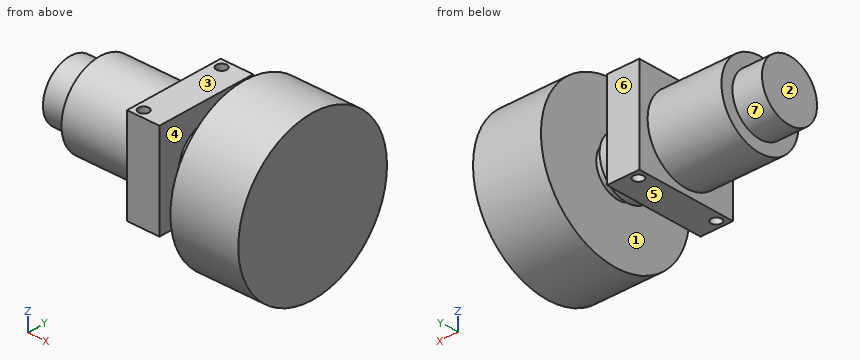
from build123d import *

# Parameters (mm, degrees)
SKETCH_R          = 14
PAD_DEPTH         = 25
SKETCH001_W       = 34
SKETCH001_H       = 32
PAD001_DEPTH      = 11
SKETCH002_R       = 10
PAD002_DEPTH      = 9
SKETCH003_R       = 8
PAD003_DEPTH      = 3
PAD004_DEPTH      = 12
SKETCH005_R       = 1.75
POCKET_DEPTH      = 100
SKETCH006_R       = 27
PAD005_DEPTH      = 12
PAD005_DEPTH_BACK = 11
SKETCH007_R       = 10
PAD006_DEPTH      = 10


with BuildPart() as part:
    # Sketch → Pad (new body)
    with BuildSketch(Plane.YZ):
        Circle(SKETCH_R)
    extrude(amount=-PAD_DEPTH)

    # Sketch001 (on Face2 of Pad) → Pad001 (join)
    with BuildSketch(Plane.YZ):
        Rectangle(SKETCH001_W, SKETCH001_H)
    extrude(amount=PAD001_DEPTH)

    # Sketch002 (on Face5 of Pad001) → Pad002 (join)
    with BuildSketch(Plane.YZ.offset(11)):
        Circle(SKETCH002_R)
    extrude(amount=PAD002_DEPTH)

    # Sketch003 (on Face10 of Pad002) → Pad003 (join)
    with BuildSketch(Plane.YZ.offset(20)):
        Circle(SKETCH003_R)
    extrude(amount=PAD003_DEPTH)

    # Sketch004 (on Face12 of Pad003) → Pad004 (join)
    with BuildSketch(Plane.YZ.offset(23)):
        Polygon((0, 4.041452), (-3.5, 2.020726), (-3.5, -2.020726), (0, -4.041452), (3.5, -2.020726), (3.5, 2.020726), align=None)
    extrude(amount=PAD004_DEPTH)

    # Sketch005 (on Face1 of Pad004) → Pocket (cut)
    with BuildSketch(Plane(origin=(0, 0, 16), x_dir=(0, -1, 0), z_dir=(0, 0, 1))):
        with Locations((-14.15, 3)):
            Circle(SKETCH005_R)
        with Locations((14.15, 3)):
            Circle(SKETCH005_R)
    extrude(amount=-POCKET_DEPTH, mode=Mode.SUBTRACT)

    # Sketch006 (on Face21 of Pocket) → Pad005 (join, two sides)
    with BuildSketch(Plane.YZ.offset(35)) as pad005_sk:
        Circle(SKETCH006_R)
    extrude(amount=PAD005_DEPTH)
    extrude(pad005_sk.sketch, amount=-PAD005_DEPTH_BACK)

    # Sketch007 (on Face11 of Pad005) → Pad006 (join)
    with BuildSketch(Plane(origin=(-25, 0, 0), x_dir=(0, 1, 0), z_dir=(-1, 0, 0))):
        Circle(SKETCH007_R)
    extrude(amount=PAD006_DEPTH)


solid = part.part
Build history of the part. All positions in model axes, mm. Face numbers are marked on the shaded views. A direction names the side the tool comes from. Give positions to 0.01 mm unless a question says otherwise; leave off trailing zeros. Order: outer loops, then holes, each group sorted by start corner. A loop starts at its lowest first (then second) coordinate and runs counter-clockwise, first axis right, second up. Notation, with made-up numbers: M 77.5,-34.75 L 101.5,-34.75 A20 ccw 101.5,-23.75 Z; hole C -18,-35 d1. An arc over 180 degrees is marked long. Put each result on its own line as item: value.
Item 1: Pull direction X, two halves, no side cores. Call the marked faces 1, 2, 3 and 4: +X half, -X half, draft (parallel to the pull), parting line (faces both ways), or undercut.
Results are:
face 1: undercut
face 2: -X half
face 3: draft
face 4: undercut
Item 2: Cut at C-C on y = 9. Write the cut outline in (x, z), then the cut area to 3 significant figures.
Results are:
outline: M -35,-4.36 L -25,-4.36 L -25,-10.72 L 0,-10.72 L 0,-16 L 11,-16 L 11,-4.36 L 20,-4.36 L 20,4.36 L 11,4.36 L 11,16 L 0,16 L 0,10.72 L -25,10.72 L -25,4.36 L -35,4.36 Z; M 24,-25.46 L 47,-25.46 L 47,25.46 L 24,25.46 Z
area: 2,220 mm2
Item 3: Drop flat-ended pins along their axis: pin 1 Ø9 at (x, y) = (8, 6.5) entering from -Z; pin 2 Ø8 at (x, z) = (29.5, -11) entering from -Y; pin 3 Ø9 at (x, y) = (6, 4.5) entering from +Z. Give the stop position or say it passes through.
Results are:
pin 1: z = -16
pin 2: y = -26.08
pin 3: z = 16
Item 4: Cut at A-A on x = 3. Write the cut outline in (y, z), then the cut area to 3 significant figures.
Results are:
outline: M -17,-16 L -15.9,-16 L -15.9,16 L -17,16 Z; M -12.4,-16 L 12.4,-16 L 12.4,16 L -12.4,16 Z; M 15.9,-16 L 17,-16 L 17,16 L 15.9,16 Z
area: 864 mm2
Item 5: Wall check: probe 1 along X at (y, z) = (14.15, 2); probe 2 along X at (y, z) = (-10, -4); probe 3 along X at (y, z) = (10, 15). Give the ranges that are in metal, low to high.
Results are:
probe 1: 0 to 1.25, 4.75 to 11, 24 to 47
probe 2: -25 to 11, 24 to 47
probe 3: 0 to 11, 24 to 47
Item 6: Cut at B-B on z = 0. Count the separate pieces of the cut face and the enclosed holes in it, then the cut area to 3 significant figures.
Results are:
separate pieces: 1
enclosed holes: 2
area: 2,730 mm2
Item 7: Which spindle directions (+Z, -Z, +X, -X, +Y, -Y) get a long thin tool onto all of the face, cutting with end or side? Do the marked faces 5, 6 and 7. Say none if no direction does.
Results are:
face 5: -Z, -X, +Y, -Y
face 6: +Z, -Z, -X, +Y
face 7: -X
Item 8: Cut at D-D on z = 5.5. Write the cut outline in (x, y), then the cut area to 3 significant figures.
Results are:
outline: M -35,-8.35 L -25,-8.35 L -25,-12.87 L 0,-12.87 L 0,-17 L 11,-17 L 11,-8.35 L 20,-8.35 L 20,-5.81 L 23,-5.81 L 23,5.81 L 20,5.81 L 20,8.35 L 11,8.35 L 11,17 L 0,17 L 0,12.87 L -25,12.87 L -25,8.35 L -35,8.35 Z; M 24,-26.43 L 47,-26.43 L 47,26.43 L 24,26.43 Z; hole C 3,-14.15 d3.5; hole C 3,14.15 d3.5
area: 2,570 mm2
